```python
from build123d import *

# Parameters (mm, degrees)
SKETCH1_W                       = 321.691
SKETCH1_H                       = 254
BASE_EXTRUDE_DEPTH              = 19.05
BOSS_EXTRUDE1_DEPTH             = 15.875
SKETCH3_W                       = 139.7
SKETCH3_H                       = 119.186428927
CUT_EXTRUDE1_DEPTH              = 15.875
FILLET3_R                       = 2.54
FILLET5_R                       = 6.35
FILLET6_R                       = 2.54
CBORE_FOR_M10_SHCS1_D           = 11
CBORE_FOR_M10_SHCS1_CBORE_D     = 18
CBORE_FOR_M10_SHCS1_CBORE_DEPTH = 10
LPATTERN1_COUNT                 = 4
LPATTERN1_PITCH                 = 50.8
CBORE_FOR_M10_SHCS2_D           = 11
CBORE_FOR_M10_SHCS2_CBORE_D     = 18
CBORE_FOR_M10_SHCS2_CBORE_DEPTH = 10
LPATTERN2_COUNT                 = 4
LPATTERN2_PITCH                 = 50.8


with BuildPart() as part:
    # Sketch1 → Base-Extrude (new body)
    with BuildSketch(Plane.XY):
        with Locations((184.326529799, 339.562514452)):
            Rectangle(SKETCH1_W, SKETCH1_H)
    extrude(amount=BASE_EXTRUDE_DEPTH)

    # Sketch2 → Boss-Extrude1 (add)
    with BuildSketch(Plane(origin=(0, 0, 0), x_dir=(-1, 0, 0), z_dir=(0, 0, -1))):
        Polygon((-273.226529799, 392.273888287), (-273.226529799, 245.776085525), (-95.426529799, 245.776085525), (-95.426529799, 392.273888287), (-105.142059927, 403.062514452), (-263.51099967, 403.062514452), align=None)
    extrude(amount=BOSS_EXTRUDE1_DEPTH)

    # Sketch3 → Cut-Extrude1 (cut)
    with BuildSketch(Plane(origin=(0, 0, -15.875), x_dir=(-1, 0, 0), z_dir=(0, 0, -1))):
        with Locations((-184.326529799, 324.419299989)):
            Rectangle(SKETCH3_W, SKETCH3_H)
    extrude(amount=-CUT_EXTRUDE1_DEPTH, mode=Mode.SUBTRACT)

    # Fillet3
    fillet3_edges = [part.edges().sort_by_distance(p)[0] for p in [
        (95.426529799, 319.024986906, 0),
        (100.284294863, 397.668201369, 0),
        (184.326529799, 403.062514452, 0),
        (268.368764734, 397.668201369, 0),
        (273.226529799, 319.024986906, 0),
        (184.326529799, 245.776085525, 0),
    ]]
    fillet(fillet3_edges, radius=FILLET3_R)

    # Fillet5
    fillet5_edges = [part.edges().sort_by_distance(p)[0] for p in [
        (254.176529799, 264.826085525, -7.9375),
        (114.476529799, 264.826085525, -7.9375),
        (114.476529799, 384.012514452, -7.9375),
        (254.176529799, 384.012514452, -7.9375),
    ]]
    fillet(fillet5_edges, radius=FILLET5_R)

    # Fillet6
    fillet6_edges = [part.edges().sort_by_distance(p)[0] for p in [
        (254.176529799, 324.419299989, 0),
        (184.326529799, 384.012514452, 0),
        (184.326529799, 264.826085525, 0),
        (114.476529799, 324.419299989, 0),
        (116.336401738, 266.685957465, 0),
        (116.336401738, 382.152642512, 0),
        (252.316657859, 266.685957465, 0),
        (252.316657859, 382.152642512, 0),
    ]]
    fillet(fillet6_edges, radius=FILLET6_R)

    # CBORE for M10 SHCS1 (through all)
    with Locations(Plane(origin=(0, 0, 0), x_dir=(-1, 0, 0), z_dir=(0, 0, -1))):
        with Locations((-312.914029799, 415.762514452)):
            cbore_for_m10_shcs1 = CounterBoreHole(CBORE_FOR_M10_SHCS1_D / 2, CBORE_FOR_M10_SHCS1_CBORE_D / 2, CBORE_FOR_M10_SHCS1_CBORE_DEPTH)

    # LPattern1: CBORE for M10 SHCS1 ×4
    with Locations(*[(0, -i * LPATTERN1_PITCH, 0) for i in range(1, LPATTERN1_COUNT)]):
        add(cbore_for_m10_shcs1, mode=Mode.SUBTRACT)

    # CBORE for M10 SHCS2 (through all)
    with Locations(Plane(origin=(0, 0, 0), x_dir=(-1, 0, 0), z_dir=(0, 0, -1))):
        with Locations((-55.739029799, 415.762514452)):
            cbore_for_m10_shcs2 = CounterBoreHole(CBORE_FOR_M10_SHCS2_D / 2, CBORE_FOR_M10_SHCS2_CBORE_D / 2, CBORE_FOR_M10_SHCS2_CBORE_DEPTH)

    # LPattern2: CBORE for M10 SHCS2 ×4
    with Locations(*[(0, -i * LPATTERN2_PITCH, 0) for i in range(1, LPATTERN2_COUNT)]):
        add(cbore_for_m10_shcs2, mode=Mode.SUBTRACT)


solid = part.part
```
Build history of the part. All positions in model axes, mm. A direction names the side the tool comes from. Coordinates: 2 decimals unless noted, no trailing zeros. Order: outer loops, then holes, each group sorted by start corner. A loop starts at its lowest first (then second) coordinate and runs counter-clockwise, first axis right, second up. Notation, with made-up numbers: M 45,-9 L 81,-9 A21 ccw 81,22 Z; hole C -33.5,57.25 d7. An arc over 180 degrees is marked long. One line per question, with ' | ' between items. Start each with the question number.
1. Cut at A-A (z = -10.5). Write the cut outline in (x, y), plus the area to 3 significant figures.
2. Wall check: line 1 along Y through (x, z) = (194, -10); line 2 along X through (y, z) = (307.5, -7); line 3 along Z through (x, y) = (322.5, 287.5). Give the ranges that are in metal, low to high. Write a range as [from, to].
3. Tool access for faces 5 (the face through (116.386, 266.637, -9.114)), 6 (the face through (345.172, 338, 9)): list every direction of +Z, -Z, +X, -X, +Y, -Y with a clear straight run to the whole face (end or side of a thin tool).
4. Cut at C-C (y = 276). Write the cut outline in (x, z) (3 decimals), plus the area to 3 significant figures.
5. Cut at B-B (x = 150). Write the cut outline in (y, z) (3 decimals).
6. Cut at D-D (x = 80). Write the cut outline in (y, z), plus the area to 3 significant figures.
7. Flat gauge pins, fed straight in: P1, Ø12, axis at x = 207.5, y = 416, coming from the -Z side; P2, Ø1, axis at x = 141, z = -11, coming from the +Y side; P3, Ø4, axis at y = 317, z = -7.5, coming from the +X side; P4, Ø9, axis at x = 312.91, y = 314.16, coming from the +Z side. Where does each tip first touch, or does it go through?
8. Mould opens along Y. For faces 1 (the face through (185, 384.013, -9)), 2 (the face through (309, 318.3, 10)), 3 (the face through (186, 256, -15.875)), 4 (the face through (268.962, 398.151, -0.724)) say: +Y half, -Y half, draft (parallel to the pull), parting line (faces both ways), or undercut.
The answers:
1) outline: M 95.43,245.78 L 273.23,245.78 L 273.23,392.27 L 263.51,403.06 L 105.14,403.06 L 95.43,392.27 Z; hole M 114.48,271.18 A6.35 ccw 120.83,264.83 L 247.83,264.83 A6.35 ccw 254.18,271.18 L 254.18,377.66 A6.35 ccw 247.83,384.01 L 120.83,384.01 A6.35 ccw 114.48,377.66 Z | area: 11,200 mm2
2) line 1: y = [245.78, 264.83], [384.01, 403.06] | line 2: x = [95.43, 114.48], [254.18, 273.23] | line 3: z = [0, 19.05]
3) face 5: -Z | face 6: +Z, -Z, +X, +Y, -Y
4) outline: M 23.481,0 L 92.887,0 A2.54 cw 95.427,-2.54 L 95.427,-15.875 L 114.477,-15.875 L 114.477,-2.54 A2.54 cw 117.017,0 L 251.637,0 A2.54 cw 254.177,-2.54 L 254.177,-15.875 L 273.227,-15.875 L 273.227,-2.54 A2.54 cw 275.767,0 L 345.172,0 L 345.172,19.05 L 23.481,19.05 Z | area: 6,740 mm2
5) outline: M 212.563,0 L 243.236,0 A2.54 cw 245.776,-2.54 L 245.776,-15.875 L 264.826,-15.875 L 264.826,-2.54 A2.54 cw 267.366,0 L 381.473,0 A2.54 cw 384.013,-2.54 L 384.013,-15.875 L 403.063,-15.875 L 403.063,-2.54 A2.54 cw 405.603,0 L 466.563,0 L 466.563,19.05 L 212.563,19.05 Z
6) outline: M 212.56,0 L 466.56,0 L 466.56,19.05 L 212.56,19.05 Z | area: 4,840 mm2
7) P1: stops at z = 0 | P2: stops at y = 403.06 | P3: stops at x = 273.23 | P4: passes through
8) face 1: undercut | face 2: undercut | face 3: draft | face 4: +Y half
